The listing builds one solid part. Answer for the finished solid, in the listing's coordinates (mm). A direction names the side the tool comes from. Give positions to 0.01 mm unless a question says otherwise; leave off trailing zeros. Loops run counter-clockwise (first coordinate to the right, second up) from the corner with the lowest first, then second, coordinate; pieces in that order, holes last.
Item 1: This flat-tipped pin is pushed along its axis until it touches: pin 1 Ø5.5 at (y, z) = (0, 0) entering from +X. Where does it stop, or does it pass through?
Item 2: A tool of negligible diameter and unlimited length cuts with its end or side. For faces 1 (the face through (30.42, 6.699, 6.715)), 2 (the face through (38, 0, 3)), from which of +Z, -Z, +X, -X, +Y, -Y can it reach the whole face along a straight path? Write none if from no direction.
Item 3: Section A-A, the plane z = 0 is taken. Give the vertices of the cut face in (x, y), and give its area (3 significant figures).
Item 4: The mould has two halves that part along Z. Classify faces 3 (the face through (16, 0, 0)), 4 (the face through (30, 7, 0)), 5 (the face through (30.42, -6.715, -6.699)): pulls with the +Z half, pulls with the -Z half, needs draft (parallel to the pull), parting line crosses it, or undercut.
Item 5: Section B-B, the plane x = 20 is taken. Give the vertices of the cut face in (y, z).
Item 6: Consider line 1 along Y through (x, z) = (35, 0); line 2 along X through (y, z) = (-2, -0.5); line 3 along Y through (x, z) = (41.5, 2.75). Determine where each line is inside the solid, lowest interval first.
from build123d import *

# Parameters (mm, degrees)
SKETCH1_W           = 14
SKETCH1_H           = 14
BOSS_EXTRUDE1_DEPTH = 60
FILLET1_R           = 1
SKETCH2_R           = 3
CUT_EXTRUDE1_DEPTH  = 44


with BuildPart() as part:
    # Sketch1 → Boss-Extrude1 (new body)
    with BuildSketch(Plane(origin=(0, 0, 0), x_dir=(0, 0, -1), z_dir=(1, 0, 0))):
        Rectangle(SKETCH1_W, SKETCH1_H)
    extrude(amount=BOSS_EXTRUDE1_DEPTH)

    # Fillet1
    fillet1_edges = [part.edges().sort_by_distance(p)[0] for p in [
        (30, -7, -7),
        (30, -7, 7),
        (30, 7, 7),
        (30, 7, -7),
    ]]
    fillet(fillet1_edges, radius=FILLET1_R)

    # Sketch2 → Cut-Extrude1 (cut)
    with BuildSketch(Plane(origin=(60, 0, 0), x_dir=(0, 0, -1), z_dir=(1, 0, 0))):
        Circle(SKETCH2_R)
    extrude(amount=-CUT_EXTRUDE1_DEPTH, mode=Mode.SUBTRACT)


solid = part.part
Worked answers:
1. pin 1: stops at x = 16
2. face 1: +Z, +X, -X, +Y
2. face 2: +X
3. outline: (0, -7) - (60, -7) - (60, -3) - (16, -3) - (16, 3) - (60, 3) - (60, 7) - (0, 7) - close
3. area: 576 mm2
4. face 3: undercut
4. face 4: needs draft
4. face 5: pulls with the -Z half
5. outline: (-7, -6) arc R1 ccw to (-6, -7) - (6, -7) arc R1 ccw to (7, -6) - (7, 6) arc R1 ccw to (6, 7) - (-6, 7) arc R1 ccw to (-7, 6) - close; hole circle Ø6 at (0, 0)
6. line 1: y = -7 to -3, 3 to 7
6. line 2: x = 0 to 16
6. line 3: y = -7 to -1.2, 1.2 to 7
